Input: part model. Units: mm. Frame: model coordinates. Face numbers are marked on the shaded views. A direction names the side the tool comes from. Give positions to 0.01 mm unless a question says otherwise; leave off trailing zeros. Order: outer loops, then holes, each group sorted by start corner. A loop starts at its lowest first (then second) coordinate and runs counter-clockwise, first axis right, second up. Notation, with made-up numbers: M 15.25,-35 L 65.25,-35 A19 cw 65.25,0 Z; hole C 20.25,42.25 d11. An arc over 180 degrees is marked long. Use a Markdown table: item, result.
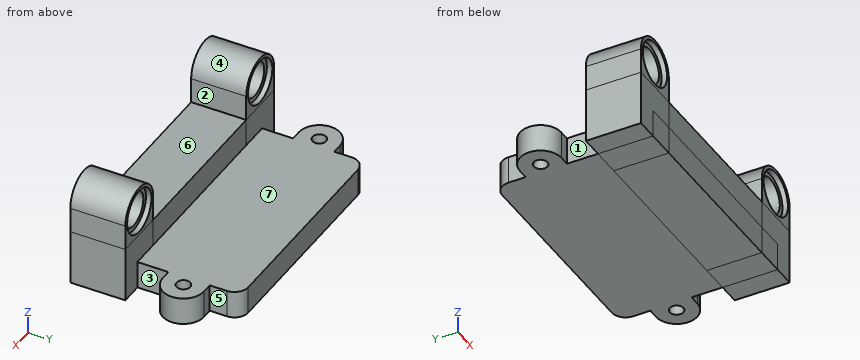
Autodesk Fusion 360 part; units mm, degrees
sketch "Sketch1" plane through (0, 0, 0) normal (0, 0, 1) x (1, 0, 0) in component "Component"
  line L0 (16.5, -7.5) -> (-16.5, -7.5)
  line L1 (-16.5, -7.5) -> (-16.5, 7.5)
  line L2 (-16.5, 7.5) -> (16.5, 7.5)
  line L3 (16.5, 7.5) -> (16.5, -7.5)
  line L4 (16.5, -7.5) -> (-16.5, 7.5) construction
  line L5 (-16.5, -7.5) -> (16.5, 7.5) construction
  line L6 (-18, 0) -> (18, 0) construction
  circle A0 centre (-18, 0) radius 1
  circle A1 centre (-18, 0) radius 1.5 construction
  circle A2 centre (18, 0) radius 1
  circle A3 centre (18, 0) radius 1.5 construction
  line L7 (-18, -3) -> (18, -3)
  arc A4 (18, -3) -> (17.9937, 3) centre (18, 0) ccw
  line L8 (17.9937, 3) -> (-18, 3)
  arc A5 (-18, 3) -> (-18, -3) centre (-18, 0) ccw
  line L9 (-18, 0) -> (18, 0) construction
  line L10 (21, 0.0031) -> (-21, 0)
  dimension "d1" = 33
  dimension "d2" = 15
  dimension "d3" = 36
  dimension "d4" = 2
  dimension "d6" = 7.5
  dimension "d7" = 2
  dimension "d31" = 42
extrude "Extrude1" add sketch "Sketch1" along normal blind 4 contours L0 L1 L3 L7 | L1 L3 L7 L10 | L3 A2 L7 A4 L10 | L1 A0 L7 A5 L10 | L1 L3 L8 L10 | L3 A2 A4 L8 L10 | L1 A0 L8 A5 L10 | L1 L2 L3 L8 in component "Component"
sketch "Sketch4" plane through (0, -7.5, 0) normal (0, -1, 0) x (1, 0, 0) in component "Component"
  line L0 (-16.5, 0) -> (16.5, 0)
  line L1 (16.5, 0) -> (16.5, 4)
  line L2 (16.5, 4) -> (-16.5, 4)
  line L3 (-16.5, 4) -> (-16.5, 0)
  circle A0 centre (-16, 11.69) radius 2.52
  circle A1 centre (-16, 11.69) radius 3.22
  line L4 (-16, 8) -> (16, 8)
  arc A2 (16, 8) -> (16, 15.38) centre (16, 11.69) ccw construction
  line L5 (16, 15.38) -> (-16, 15.38) construction
  arc A3 (-16, 15.38) -> (-16, 8) centre (-16, 11.69) ccw construction
  line L6 (-16, 11.69) -> (16, 11.69) construction
  line L7 (-21, 0) -> (21, 0)
  line L8 (21, 0) -> (21, 8)
  line L9 (21, 8) -> (-21, 8)
  line L10 (-21, 8) -> (-21, 0)
  line L11 (-19.69, 11.69) -> (-19.69, 0)
  line L12 (19.69, 11.69) -> (19.69, 0)
  circle A4 centre (-16, 11.69) radius 3.69 construction
  line L13 (-12.31, 11.69) -> (-12.31, -0.0046)
  circle A5 centre (16, 11.69) radius 3.69 construction
  line L14 (12.31, 11.69) -> (12.31, -0.001)
  arc A6 (19.69, 11.69) -> (12.31, 11.69) centre (16, 11.69) ccw
  arc A7 (-12.31, 11.69) -> (-19.69, 11.69) centre (-16, 11.69) ccw
  dimension "d23" = 5.04
  dimension "d24" = 6.44
  dimension "d27" = 7.38
  dimension "d29" = 42
  dimension "d30" = 8
  dimension "d32" = 32
  dimension "d33" = 7.38
  dimension "d34" = 7.38
extrude "Extrude2" add sketch "Sketch4" along normal blind 8 contours L0 L1 L2 L7 L14 | L0 L2 L7 L13 L14 | L1 L2 L4 L7 L9 L12 L14 | L0 L2 L3 L7 L13 | L2 L4 L9 L13 L14 | L7 L8 L9 L12 | L2 L3 L4 L7 L9 L11 L13 | L4 L9 L12 L14 A6 | L7 L9 L10 L11 | L4 L9 L11 L13 A7 | A0 | A1 in component "Component"
extrude "Extrude3" cut sketch "Sketch4" along normal blind 8 contours A0 in component "Component"
extrude "Extrude4" cut sketch "Sketch4" along normal blind 0.8 contours A1 in component "Component"
ref_plane "WorkPlane1" through (-16, -11.5, 11.69) normal (0, -1, 0) x (1, 0, 0) in component "Component"
mirror "Mirror1" about plane through (-16, -11.5, 11.69) normal (0, -1, 0) of "Extrude4" in component "Component"
ref_plane "WorkPlane2" through (0, -11.5, 4) normal (1, 0, 0) x (0, 0, 1) in component "Component"
mirror "Mirror2" about plane through (0, -11.5, 4) normal (1, 0, 0) of "Extrude3", "Extrude4", "Mirror1" in component "Component"
extrude "Extrude5" cut 2 faces at (20.1267, -12.8333, 8) (-20.1267, -10.1667, 8) along direction (0, 0, -1) blind 8 in component "Component"
fillet "Fillet1" radius 2 2 edges at (-16.5, 7.5, 2) (16.5, 7.5, 2) in component "Component"
component "Component" placed x (1, 0, 0) y (0, 1, 0) z (0, 0, 1) at (0, 0, 0)
equation "d23 = 4.8 mm + 0.24 mm"
equation "d24 = 6.2 mm + 0.24 mm"
1) Mould query, pull axis X, two halves, no side actions, for the marked faces 1, 2, 3 and 4. Classes: released by +X, released by -X, zero draft, split by the parting line, or undercut.
Response values:
| item | result |
|---|---|
| face 1 | released by -X |
| face 2 | undercut |
| face 3 | released by +X |
| face 4 | undercut |
2) Material intervals for line 1 (Y direction, x = -18, z = 1.7); line 2 (X direction, y = 0, z = 0.8); line 3 (Z direction, x = 16, y = -13), sorted ascending. Write a range as from..to.
Response values:
| item | result |
|---|---|
| line 1 | y = -15.5..-7.5, -3..-1, 1..3 |
| line 2 | x = -21..-19, -17..17, 19..21 |
| line 3 | z = 0..9.17, 14.21..15.38 |
3) Cut plane B-B on z = 2.75. Return loops of the section in (x, y), and give its area (3 significant figures).
Response values:
| item | result |
|---|---|
| outline | M -19.69,-15.5 L 19.69,-15.5 L 19.69,-7.5 L 16.5,-7.5 L 16.5,-3 L 18,-3 A3 ccw 17.99,3 L 16.5,3 L 16.5,5.5 A2 ccw 14.5,7.5 L -14.5,7.5 A2 ccw -16.5,5.5 L -16.5,3 L -18,3 A3 ccw -18,-3 L -16.5,-3 L -16.5,-7.5 L -19.69,-7.5 Z; hole C -18,0 d2; hole C 18,0 d2 |
| area | 848 mm² |
4) First-contact query: pin 1 Ø1.2 at (x, y) = (18, 0) entering from +Z; pin 2 Ø6 at (x, z) = (16, 11.69) entering from +Y; pin 3 Ø4 at (y, z) = (-10, 3.5) entering from +X; pin 4 Ø3 at (x, y) = (-18, 0) entering from +Z. Flat tips, straight axial feed; report the tip coordinate or a pass-through.
Response values:
| item | result |
|---|---|
| pin 1 | passes through |
| pin 2 | stops at y = -8.3 |
| pin 3 | stops at x = 19.69 |
| pin 4 | stops at z = 4 |
5) Cut plane D-D on x = 16. Return loops of the section in (y, z).
Response values:
| item | result |
|---|---|
| outline | M -15.5,0 L 6.82,0 L 6.82,4 L -7.5,4 L -7.5,8.47 L -8.3,8.47 L -8.3,9.17 L -14.7,9.17 L -14.7,8.47 L -15.5,8.47 Z; M -15.5,14.91 L -14.7,14.91 L -14.7,14.21 L -8.3,14.21 L -8.3,14.91 L -7.5,14.91 L -7.5,15.38 L -15.5,15.38 Z |
6) Cut plane A-A on y = 0. Return loops of the section in (x, z), and give its area (3 significant figures).
Response values:
| item | result |
|---|---|
| outline | M -21,0 L -19,0 L -19,4 L -21,4 Z; M -17,0 L 17,0 L 17,4 L -17,4 Z; M 19,0 L 21,0 L 21,4 L 19,4 Z |
| area | 152 mm² |
7) Reachability of the marked faces 5, 6 and 7 from +Z, -Z, +X, -X, +Y, -Y: full face, straight path, thin tool, end or side. Return the list, or none.
Response values:
| item | result |
|---|---|
| face 5 | +Z, -Z, +X, +Y |
| face 6 | +Z, +Y, -Y |
| face 7 | +Z, +X, -X, +Y |
8) Cut plane C-C on y = -11.25. Return loops of the section in (x, z), and give its area (3 significant figures).
Response values:
| item | result |
|---|---|
| outline | M -19.69,0 L 19.69,0 L 19.69,11.69 A3.69 ccw 12.31,11.69 L 12.31,8 L -12.31,8 L -12.31,11.69 A3.69 ccw -19.69,11.69 Z; hole C -16,11.69 d5.04; hole C 16,11.69 d5.04 |
| area | 372 mm² |
